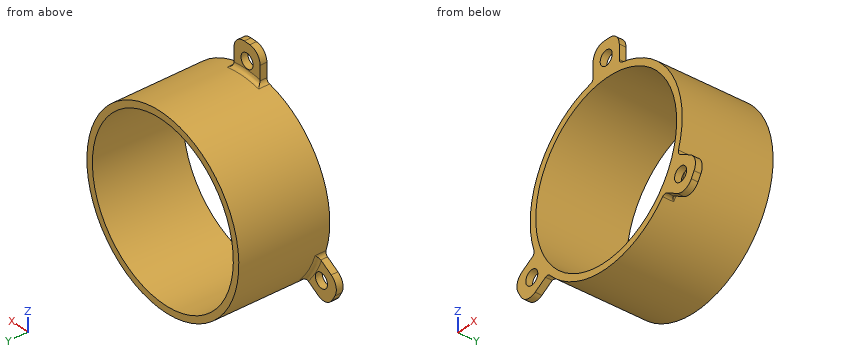
```python
from build123d import *

# Parameters (mm, degrees)
SKETCH1_R           = 20.5
BOSS_EXTRUDE2_DEPTH = 20
SHELL1_T            = 1.6
CUT_EXTRUDE1_START  = -10
SKETCH7_R           = 20.5
CUT_EXTRUDE1_DEPTH  = 10
SKETCH8_R           = 1.75
BOSS_EXTRUDE3_DEPTH = 1.6
FILLET1_R           = 1


with BuildPart() as part:
    # Sketch1 → Boss-Extrude2 (new body)
    with BuildSketch(Plane(origin=(0, 0, 0), x_dir=(1, 0, 0), z_dir=(0, 1, 0))):
        with Locations(Location((0, 0, 0), (0, 0, 270))):
            Circle(SKETCH1_R)
    extrude(amount=BOSS_EXTRUDE2_DEPTH)

    # Shell1
    shell1_openings = [part.faces().sort_by_distance(p)[0] for p in [
        (0, 20, 0),
    ]]
    offset(amount=SHELL1_T, openings=shell1_openings, kind=Kind.INTERSECTION)

    # Sketch7 → Cut-Extrude1 (cut)
    with BuildSketch(Plane(origin=(0, 0, 0), x_dir=(1, 0, 0), z_dir=(0, 1, 0)).offset(CUT_EXTRUDE1_START)):
        with Locations(Location((0, 0, 0), (0, 0, 270))):
            Circle(SKETCH7_R)
    extrude(amount=CUT_EXTRUDE1_DEPTH, mode=Mode.SUBTRACT)

    # Sketch8 → Boss-Extrude3 (add)
    # profile 1 of 3: a face of its own
    with BuildSketch(Plane(origin=(0, 0, 0), x_dir=(1, 0, 0), z_dir=(0, 1, 0))):
        with BuildLine():
            Line((-3.803893319, -20.862908404), (-3.803893319, -26.062908404))
            ThreePointArc((-3.803893319, -26.062908404), (-2.925213663, -28.184228747), (-0.803893319, -29.062908404))
            Line((-0.803893319, -29.062908404), (0.803893319, -29.062908404))
            ThreePointArc((0.803893319, -29.062908404), (2.925213663, -28.184228747), (3.803893319, -26.062908404))
            Line((3.803893319, -26.062908404), (3.803893319, -20.862908404))
            ThreePointArc((3.803893319, -20.862908404), (0, -21.291513217), (-3.803893319, -20.862908404))
        make_face()
        with Locations(Location((0, -25, 0), (0, 0, 270))):
            Circle(SKETCH8_R, mode=Mode.SUBTRACT)
    # profile 2 of 3: a face of its own
    with BuildSketch(Plane(origin=(0, 0, 0), x_dir=(1, 0, 0), z_dir=(0, 1, 0))):
        with BuildLine():
            Line((-16.165862015, 13.725722449), (-20.669194115, 16.325722449))
            ThreePointArc((-20.669194115, 16.325722449), (-22.94565125, 16.625423717), (-24.767270326, 15.227646238))
            Line((-24.767270326, 15.227646238), (-25.571163645, 13.835262166))
            ThreePointArc((-25.571163645, 13.835262166), (-25.870864913, 11.55880503), (-24.473087434, 9.737185954))
            Line((-24.473087434, 9.737185954), (-19.969755334, 7.137185954))
            ThreePointArc((-19.969755334, 7.137185954), (-18.438991331, 10.645756608), (-16.165862015, 13.725722449))
        make_face()
        with Locations(Location((-21.650635095, 12.5, 0), (0, 0, 270))):
            Circle(SKETCH8_R, mode=Mode.SUBTRACT)
    # profile 3 of 3: a face of its own
    with BuildSketch(Plane(origin=(0, 0, 0), x_dir=(1, 0, 0), z_dir=(0, 1, 0))):
        with BuildLine():
            Line((19.969755334, 7.137185954), (24.473087434, 9.737185954))
            ThreePointArc((24.473087434, 9.737185954), (25.870864913, 11.55880503), (25.571163645, 13.835262166))
            Line((25.571163645, 13.835262166), (24.767270326, 15.227646238))
            ThreePointArc((24.767270326, 15.227646238), (22.94565125, 16.625423717), (20.669194115, 16.325722449))
            Line((20.669194115, 16.325722449), (16.165862015, 13.725722449))
            ThreePointArc((16.165862015, 13.725722449), (18.438991331, 10.645756608), (19.969755334, 7.137185954))
        make_face()
        with Locations(Location((21.650635095, 12.5, 0), (0, 0, 270))):
            Circle(SKETCH8_R, mode=Mode.SUBTRACT)
    extrude(amount=-BOSS_EXTRUDE3_DEPTH)

    # Fillet1
    fillet1_edges = [part.edges().sort_by_distance(p)[0] for p in [
        (1.909082947, 0, 22.017388635),
        (-3.803893319, -0.8, 21.770172154),
        (3.803893319, -0.8, 21.770172154),
        (-19.139161424, 0, -11.05),
        (-16.951575471, -0.8, -14.179354325),
        (-20.75546879, -0.8, -7.590817829),
        (19.139161424, 0, -11.05),
        (20.75546879, -0.8, -7.590817829),
        (16.951575471, -0.8, -14.179354325),
    ]]
    fillet(fillet1_edges, radius=FILLET1_R)


solid = part.part
```
Input: part model. Units: mm. Frame: model coordinates. Give positions to 0.01 mm unless a question says otherwise; leave off trailing zeros. Loops run counter-clockwise (first coordinate to the right, second up) from the corner with the lowest first, then second, coordinate; pieces in that order, holes last.
1) Line query: L1, parallel to X at y = -0.9, z = -12.5; L2, parallel to Z at x = 0, y = 8; L3, parallel to X at y = -1.25, z = 25. Output: solid intervals per line, ascending.
A:
L1: x = -25.97 to -23.4, -19.9 to -16.25, 16.25 to 19.9, 23.4 to 25.97
L2: z = -22.1 to -20.5, 20.5 to 22.1
L3: x = -3.8 to -1.75, 1.75 to 3.8
2) Section query C-C on x = 12. Return the cut outline in (y, z), and give its area (3 significant figures).
A:
outline: (-1.6, -18.56) - (20, -18.56) - (20, -16.62) - (-1.6, -16.62) - close; (-1.6, 16.62) - (20, 16.62) - (20, 18.56) - (-1.6, 18.56) - close
area: 83.7 mm2
3) Section query A-A on x = 0. Return the cut outline in (y, z), and give its area (3 significant figures).
A:
outline: (-1.6, -22.1) - (20, -22.1) - (20, -20.5) - (-1.6, -20.5) - close; (-1.6, 20.5) - (20, 20.5) - (20, 22.1) - (1, 22.1) arc R1 cw to (0, 23.1) - (0, 23.25) - (-1.6, 23.25) - close; (-1.6, 26.75) - (0, 26.75) - (0, 29.06) - (-1.6, 29.06) - close
area: 74.9 mm2
4) Contact query for flat-ended pins moving along their axis: pin 1 (8 mm diameter, centred on x = 17, y = 2.5, fed in from -Z); pin 2 (2.5 mm diameter, centred on x = -20, z = -12.5, fed in from +Y); pin 3 (2 mm diameter, centred on x = -4, y = 7, fed in from +Z). Output: stop coordinate, or through.
A:
pin 1: stops at z = -17.87
pin 2: stops at y = 0.36
pin 3: stops at z = 21.9
5) Section query D-D on y = 14.75. Return the cut outline in (x, z), and give its area (3 significant figures).
A:
outline: circle Ø44.2 at (0, 0); hole circle Ø41 at (0, 0)
area: 214 mm2
6) Section query B-B on z = 0. Return the cut outline in (x, y).
A:
outline: (-22.1, -1.6) - (-20.5, -1.6) - (-20.5, 20) - (-22.1, 20) - close; (20.5, -1.6) - (22.1, -1.6) - (22.1, 20) - (20.5, 20) - close
